Geometry check sheet. Reference: the model listing, model coordinates, mm. Face numbers are marked on the shaded views. A direction names the side the tool comes from. Coordinates: 2 decimals unless noted, no trailing zeros. Write each loop counter-clockwise with the first axis right and the second up, starting at its lowest first coordinate (ties: lowest second). Pieces come first, ordered by that corner, then holes. Notation, with made-up numbers: M 42.5,84 L 50.5,84 A23 ccw 50.5,119 Z; hole C 67.25,-17.5 d6. An arc over 180 degrees is marked long. Write each question's results on one line, items separated by ' | '.
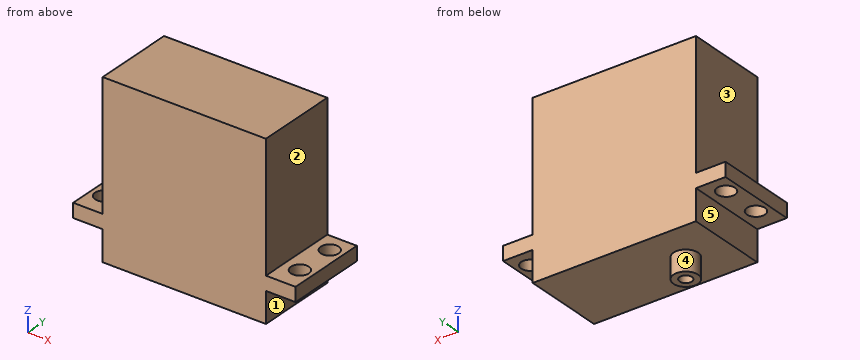
```python
from build123d import *

# Parameters (mm, degrees)
SKETCH_1_W          = 40
SKETCH_1_H          = 42
EXTRUDE_1_DEPTH     = 20
SKETCH_2_W          = 3.463290034
SKETCH_2_H          = 20
EXTRUDE_2_DEPTH     = 7.25
SKETCH_3_R          = 2.2
CUT_EXTRUDE_1_DEPTH = 7.25
SKETCH_4_R          = 3
EXTRUDE_3_DEPTH     = 5
SKETCH_5_R          = 1.5
CUT_EXTRUDE_2_DEPTH = 5


with BuildPart() as part:
    # Эскиз1 → Бобышка-Вытянуть1 (new body)
    with BuildSketch(Plane(origin=(0, 0, 0), x_dir=(1, 0, 0), z_dir=(0, 1, 0))):
        Rectangle(SKETCH_1_W, SKETCH_1_H)
    extrude(amount=EXTRUDE_1_DEPTH)

    # Эскиз2 → Бобышка-Вытянуть2 (add)
    with BuildSketch(Plane(origin=(20, 0, 0), x_dir=(0, 0, -1), z_dir=(1, 0, 0))):
        with Locations((11.768354983, 10)):
            Rectangle(SKETCH_2_W, SKETCH_2_H)
    extrude_2 = extrude(amount=EXTRUDE_2_DEPTH)

    # Эскиз3 → Вырез-Вытянуть1 (cut)
    with BuildSketch(Plane(origin=(0, 0, -13.5), x_dir=(-1, 0, 0), z_dir=(0, 0, -1))):
        with Locations((-24, 15.5)):
            Circle(SKETCH_3_R)
        with Locations((-24, 5.75)):
            Circle(SKETCH_3_R)
    cut_extrude_1 = extrude(amount=-CUT_EXTRUDE_1_DEPTH, mode=Mode.SUBTRACT)

    # Зеркальное отражение2: Бобышка-Вытянуть2, Вырез-Вытянуть1 across plane
    add(extrude_2.mirror(Plane.ZY))
    add(cut_extrude_1.mirror(Plane.ZY), mode=Mode.SUBTRACT)

    # Эскиз4 → Бобышка-Вытянуть3 (add)
    with BuildSketch(Plane(origin=(0, 0, -21), x_dir=(-1, 0, 0), z_dir=(0, 0, -1))):
        with Locations(Location((10, 10, 0), (0, 0, 180))):
            Circle(SKETCH_4_R)
    extrude(amount=EXTRUDE_3_DEPTH)

    # Эскиз5 → Вырез-Вытянуть2 (cut)
    with BuildSketch(Plane(origin=(0, 0, -26), x_dir=(-1, 0, 0), z_dir=(0, 0, -1))):
        with Locations((10, 10)):
            Circle(SKETCH_5_R)
    extrude(amount=-CUT_EXTRUDE_2_DEPTH, mode=Mode.SUBTRACT)


solid = part.part
```
Q1. Sectioned sample at A-A on x = 24. Record the cut outline in (y, z), and give its area (3 significant figures).
Geometry check:
outline: M 0,-13.5 L 3.55,-13.5 L 3.55,-10.04 L 0,-10.04 Z; M 7.95,-13.5 L 13.3,-13.5 L 13.3,-10.04 L 7.95,-10.04 Z; M 17.7,-13.5 L 20,-13.5 L 20,-10.04 L 17.7,-10.04 Z | area: 38.8 mm2
Q2. Scan lines: probe 1 along Y at (x, z) = (-24, -12); probe 2 along Y at (x, z) = (-10, -24); probe 3 along Z at (x, y) = (14.5, 5). Record each from-to range of solid material in increasing order.
Geometry check:
probe 1: y = 0 to 3.55, 7.95 to 13.3, 17.7 to 20 | probe 2: y = 7 to 8.5, 11.5 to 13 | probe 3: z = -21 to 21
Q3. Depth check by flat-ended pin: P1, Ø5, axis at x = -24, y = 15.5, coming from the +Z side; P2, Ø1, axis at x = 21, y = 7, coming from the -Z side; P3, Ø2, axis at y = 11.5, z = -7.5, coming from the -X side. Enter the tip coordinate at first touch or a pass-through.
Geometry check:
P1: stops at z = -10.04 | P2: stops at z = -13.5 | P3: stops at x = -20
Q4. Sectioned sample at B-B on y = 15.5. Record the cut outline in (x, z).
Geometry check:
outline: M -27.25,-13.5 L -26.2,-13.5 L -26.2,-10.04 L -27.25,-10.04 Z; M -21.8,-13.5 L -20,-13.5 L -20,-21 L 20,-21 L 20,-13.5 L 21.8,-13.5 L 21.8,-10.04 L 20,-10.04 L 20,21 L -20,21 L -20,-10.04 L -21.8,-10.04 Z; M 26.2,-13.5 L 27.25,-13.5 L 27.25,-10.04 L 26.2,-10.04 Z
Q5. Sectioned sample at D-D on y = 10. Record the cut outline in (x, z), and give its area (3 significant figures).
Geometry check:
outline: M -27.25,-13.5 L -20,-13.5 L -20,-21 L -13,-21 L -13,-26 L -11.5,-26 L -11.5,-21 L -8.5,-21 L -8.5,-26 L -7,-26 L -7,-21 L 20,-21 L 20,-13.5 L 27.25,-13.5 L 27.25,-10.04 L 20,-10.04 L 20,21 L -20,21 L -20,-10.04 L -27.25,-10.04 Z | area: 1,750 mm2
Q6. Access from +Z, -Z, +X, -X, +Y, -Y to the whole of each face (thin tool, end or side, straight path). Record for the marked faces 1, 2, 3, 4 and 5.
Geometry check:
face 1: -Z, +X, +Y, -Y | face 2: +Z, +X, +Y, -Y | face 3: +Z, -X, +Y, -Y | face 4: -Z | face 5: -Z, -X, +Y, -Y
Q7. Sectioned sample at C-C on x = -10. Record the cut outline in (y, z), and give its area (3 significant figures).
Geometry check:
outline: M 0,-21 L 7,-21 L 7,-26 L 8.5,-26 L 8.5,-21 L 11.5,-21 L 11.5,-26 L 13,-26 L 13,-21 L 20,-21 L 20,21 L 0,21 Z | area: 855 mm2
